Autodesk Inventor part; units mm, degrees
ref_plane "YZ Plane" through (0, 0, 0) normal (1, 0, 0) x (0, 1, 0)
ref_plane "XZ Plane" through (0, 0, 0) normal (0, 1, 0) x (-1, 0, 0)
ref_plane "XY Plane" through (0, 0, 0) normal (0, 0, 1) x (1, 0, 0)
sketch "Sketch1" plane through (0, 0, 0) normal (0, 0, 1) x (1, 0, 0)
  circle A0 centre (0, 0) radius 16
  dimension "d0" = 32
extrude "Extrusion1" add sketch "Sketch1" against normal blind 35
sketch "Sketch2" plane through (0, 0, -35) normal (0, 0, -1) x (-1, 0, 0)
  circle A0 centre (0, 0) radius 15
  dimension "d3" = 30
extrude "Extrusion2" add sketch "Sketch2" along normal blind 38
sketch "Sketch3" plane through (0, 0, -73) normal (0, 0, -1) x (-1, 0, 0)
  circle A0 centre (0, 0) radius 4.064
extrude "Extrusion3" add sketch "Sketch3" along normal blind 3
sketch "Sketch4" plane through (0, 0, 0) normal (0, 0, 1) x (1, 0, 0)
  point P0 (0, 0)
sketch "Sketch5" plane through (0, 0, 0) normal (0, 0, 1) x (1, 0, 0)
  circle A0 centre (-10.5, 0) radius 4.5
  circle A1 centre (0, 0) radius 15
  circle A2 centre (5.7991, 0) radius 4.5
  dimension "d8" = 9
extrude "Extrusion4" add sketch "Sketch5" along normal blind 13 contours A0 | A2
sketch "Sketch6" plane through (-10.5, 0, 13) normal (0, 0, 1) x (1, 0, 0)
  arc A0 (2.1608, 3.1628) -> (2.1608, -3.1628) centre (0, 0) ccw
  circle A1 centre (16.2991, 0) radius 4.5
  arc A2 (14.1383, -3.1628) -> (14.1383, 3.1628) centre (16.2991, 0) ccw
  circle A3 centre (0, 0) radius 4.5
  line L0 (14.1383, 3.1628) -> (14.1383, -3.1628)
  line L1 (2.1608, 3.1628) -> (2.1608, -3.1628)
  point P0 (10.5, 0)
extrude "Extrusion5" cut sketch "Sketch6" against normal blind 13 contours L1 A0 | L0 A2
sketch "Sketch7" plane through (0, 0, 0) normal (0, 0, 1) x (1, 0, 0)
  circle A0 centre (0, 0) radius 16
  circle A1 centre (-8.3308, 13.6601) radius 3.5
  line L0 (0, -22.632) -> (0, 23.7921)
  circle A2 centre (8.3308, 13.6601) radius 3.5
  line L1 (-22.4, 0) -> (22.4, 0)
  circle A3 centre (-8.3308, -13.6601) radius 3.5
  circle A4 centre (8.3308, -13.6601) radius 3.5
  dimension "d14" = 7
extrude "Extrusion6" add sketch "Sketch7" against normal blind 24 contours A2 A0 | A0 A2 | A4 A0 | A0 A4 | A3 A0 | A0 A3 | A1 A0 | A0 A1
properties part number "pump"
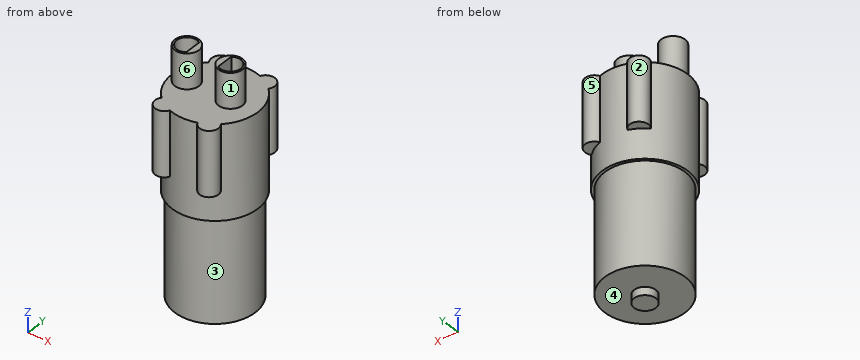
Verification items for the finished model (mm, model axes). Face numbers are marked on the shaded views. A direction names the side the tool comes from. Give positions to 0.01 mm unless a question says otherwise; leave off trailing zeros. Write each loop counter-clockwise with the first axis right and the second up, starting at its lowest first coordinate (ties: lowest second). Pieces come first, ordered by that corner, then holes. Notation, with made-up numbers: (3, 50.5) - (50, 50.5) arc R23 ccw to (50, 63.5) - close; hole circle Ø7 at (26.5, 17.5). An arc over 180 degrees is marked (long way). Put each result on its own line as item: value.
Q1. Section check D-D on x = 8.5. Record the cut outline in (y, z), and give its area (3 significant figures).
Result:
outline: (-17.16, -24) - (-13.56, -24) - (-13.56, -35) - (-12.36, -35) - (-12.36, -73) - (12.36, -73) - (12.36, -35) - (13.56, -35) - (13.56, -24) - (17.16, -24) - (17.16, 0) - (3.6, 0) - (3.6, 13) - (2.72, 13) - (2.72, 0) - (-2.72, 0) - (-2.72, 13) - (-3.6, 13) - (-3.6, 0) - (-17.16, 0) - close
area: 2,080 mm2
Q2. Scan lines: probe 1 along Z at (x, y) = (-7, 3); probe 2 along Y at (x, z) = (-10.5, 9.75); probe 3 along Y at (x, z) = (11.5, -20). Record each from-to range of solid material in increasing order. Write a range as from..to.
Result:
probe 1: -73..0
probe 2: -4.5..-3.83, 3.83..4.5
probe 3: -15.15..-12.17, -11.12..11.12, 12.17..15.15
Q3. Section check C-C on z = -13. Record the cut outline in (x, y).
Result:
outline: (-11.1, -11.52) arc R3.5 ccw (long way) to (-5.16, -15.14) arc R16 ccw to (5.16, -15.14) arc R3.5 ccw (long way) to (11.1, -11.52) arc R16 ccw to (11.1, 11.52) arc R3.5 ccw (long way) to (5.16, 15.14) arc R16 ccw to (-5.16, 15.14) arc R3.5 ccw (long way) to (-11.1, 11.52) arc R16 ccw to start
Q4. Depth check by flat-ended pin: P1, Ø12, axis at y = -8.5, z = 1, coming from the -X side; P2, Ø3, axis at x = 8, y = -0.5, coming from the +Z side; P3, Ø6, axis at y = -8.5, z = -23, coming from the -X side (3 decimals). Enter the tip coordinate at first touch or a pass-through.
Result:
P1: x = -15.79
P2: z = 0
P3: x = -15.025
Q5. Section check A-A on x = 0. Record the cut outline in (y, z), and give its area (3 significant figures).
Result:
outline: (-16, -35) - (-15, -35) - (-15, -73) - (-4.06, -73) - (-4.06, -76) - (4.06, -76) - (4.06, -73) - (15, -73) - (15, -35) - (16, -35) - (16, 0) - (-16, 0) - close
area: 2,280 mm2
Q6. Mould release check, pull along Y, two halves, no side actions. Record for the marked faces 4, 5 and 6: released by +Y, released by -Y, zero draft, split by the parting line, or undercut.
Result:
face 4: zero draft
face 5: undercut
face 6: split by the parting line
Q7. Section check B-B on y = 0. Record the cut outline in (x, z), and give its area (3 significant figures).
Result:
outline: (-16, -35) - (-15, -35) - (-15, -73) - (-4.06, -73) - (-4.06, -76) - (4.06, -76) - (4.06, -73) - (15, -73) - (15, -35) - (16, -35) - (16, 0) - (10.3, 0) - (10.3, 13) - (9.63, 13) - (9.63, 0) - (3.64, 0) - (3.64, 13) - (1.3, 13) - (1.3, 0) - (-6, 0) - (-6, 13) - (-8.34, 13) - (-8.34, 0) - (-14.33, 0) - (-14.33, 13) - (-15, 13) - (-15, 0) - (-16, 0) - close
area: 2,360 mm2
Q8. Set-up check for the marked faces 1, 2 and 3: record each of +Z, -Z, +X, -X, +Y, -Y from which the full face is reachable in a straight line by a thin tool's end or side.
Result:
face 1: +Z
face 2: +Z, -Z
face 3: -Z
